from build123d import *

# Parameters (mm, degrees)
SKETCH1_R               = 21.25
SKETCH1_R_2             = 4.2
SKETCH1_R_3             = 2.9
BOSS_EXTRUDE1_DEPTH     = 2
CUT_EXTRUDE1_DEPTH      = 171.89177862
CUT_EXTRUDE1_DEPTH_BACK = 171.89177862
SKETCH2_W               = 15
SKETCH2_H               = 2


with BuildPart() as part:
    # Sketch1 → Boss-Extrude1 (new body)
    with BuildSketch(Plane.XY):
        Polygon((-158, -56), (-146.5, -56), (-146.5, -60), (-131.5, -60), (-131.5, -56), (-106.5, -56), (-106.5, -60), (-91.5, -60), (-91.5, -56), (-66.5, -56), (-66.5, -60), (-51.5, -60), (-51.5, -56), (-26.5, -56), (-26.5, -60), (-11.5, -60), (-11.5, -56), (11.5, -56), (11.5, -60), (26.5, -60), (26.5, -56), (51.5, -56), (51.5, -60), (66.5, -60), (66.5, -56), (91.5, -56), (91.5, -60), (106.5, -60), (106.5, -56), (131.5, -56), (131.5, -60), (146.5, -60), (146.5, -56), (158, -56), (158, -24), (160, -24), (160, -4), (158, -4), (158, 16), (160, 16), (160, 36), (158, 36), (158, 56), (146.5, 56), (146.5, 58), (131.5, 58), (131.5, 56), (106.5, 56), (106.5, 58), (91.5, 58), (91.5, 56), (66.5, 56), (66.5, 58), (51.5, 58), (51.5, 56), (26.5, 56), (26.5, 58), (11.5, 58), (11.5, 56), (-11.5, 56), (-11.5, 58), (-26.5, 58), (-26.5, 56), (-51.5, 56), (-51.5, 58), (-66.5, 58), (-66.5, 56), (-91.5, 56), (-91.5, 58), (-106.5, 58), (-106.5, 56), (-131.5, 56), (-131.5, 58), (-146.5, 58), (-146.5, 56), (-158, 56), (-158, 36), (-160, 36), (-160, 16), (-158, 16), (-158, -4), (-160, -4), (-160, -24), (-158, -24), align=None)
        with Locations((10.5, -18)):
            Circle(SKETCH1_R, mode=Mode.SUBTRACT)
        with Locations((-29, -18)):
            Circle(SKETCH1_R_2, mode=Mode.SUBTRACT)
        with Locations((50, -18)):
            Circle(SKETCH1_R_2, mode=Mode.SUBTRACT)
        with Locations((-125, -40)):
            Circle(SKETCH1_R_3, mode=Mode.SUBTRACT)
        with Locations((-71, -40)):
            Circle(SKETCH1_R_3, mode=Mode.SUBTRACT)
        with Locations((-125, 12)):
            Circle(SKETCH1_R_3, mode=Mode.SUBTRACT)
        with Locations((-71, 12)):
            Circle(SKETCH1_R_3, mode=Mode.SUBTRACT)
        with BuildLine():
            Line((-93.5, -14.916994756), (-93.5, -13.083005244))
            ThreePointArc((-93.5, -13.083005244), (-94.924535841, 8.581133525), (-107.310612225, -9.25))
            Line((-107.310612225, -9.25), (-112.7, -9.25))
            Line((-112.7, -9.25), (-112.7, -18.75))
            Line((-112.7, -18.75), (-107.310612225, -18.75))
            ThreePointArc((-107.310612225, -18.75), (-94.924535841, -36.581133525), (-93.5, -14.916994756))
        make_face(mode=Mode.SUBTRACT)
    extrude(amount=BOSS_EXTRUDE1_DEPTH)

    # Sketch2 → Cut-Extrude1 (cut, two sides: drawn at the far end of the back side and taken through both)
    with BuildSketch(Plane.XY.offset(2).offset(-CUT_EXTRUDE1_DEPTH_BACK)):
        with Locations((-139, 57)):
            Rectangle(SKETCH2_W, SKETCH2_H)
        with Locations((-99, 57)):
            Rectangle(SKETCH2_W, SKETCH2_H)
        with Locations((-59, 57)):
            Rectangle(SKETCH2_W, SKETCH2_H)
        with Locations((-19, 57)):
            Rectangle(SKETCH2_W, SKETCH2_H)
        with Locations((19, 57)):
            Rectangle(SKETCH2_W, SKETCH2_H)
        with Locations((59, 57)):
            Rectangle(SKETCH2_W, SKETCH2_H)
        with Locations((99, 57)):
            Rectangle(SKETCH2_W, SKETCH2_H)
        with Locations((139, 57)):
            Rectangle(SKETCH2_W, SKETCH2_H)
    extrude(amount=CUT_EXTRUDE1_DEPTH + CUT_EXTRUDE1_DEPTH_BACK, mode=Mode.SUBTRACT)


solid = part.part
Part model, mm, in its own coordinate system. Coordinates: 2 decimals unless noted, no trailing zeros. Loops run counter-clockwise (first coordinate to the right, second up) from the corner with the lowest first, then second, coordinate; pieces in that order, holes last. Notation, with made-up numbers: (72.5, -17) -> (91.5, -17) arc R11 ccw to (91.5, -10) -> close; hole circle Ø1 at (-15.75, -24). An arc over 180 degrees is marked (long way). Use a Markdown table: item, result. Add a question column.
Item 1: Band-saw the part on C-C on z = 1.3. Give the number of separate pieces and of enclosed holes in the cut face, plus the area to 3 significant figures.
Item 2: Probe probe 1 along Y at (x, z) = (-71, 0.9); probe 2 along X at (y, z) = (-34.5, 0.1); probe 3 along Y at (x, z) = (10.5, 1.45). List the from-to ranges inside material, lowest first.
Item 3: Band-saw the part on B-B on x = 75. Write the cut outline in (y, z).
Item 4: Flat gauge pins, fed straight in: P1, Ø1, axis at y = -57.5, z = 1, coming from the +X side; P2, Ø0.6, axis at y = -58, z = 1, coming from the -X side; P3, Ø0.6, axis at y = 10.5, z = 1, coming from the +X side. Where does each tip first touch, or does it go through?
Item 5: Pull direction Y, two halves, no side cores. Call faces 1 (the cylindrical face through (-73.1, 14, 1)), 2 (the flat face through (-2, 12, 2)): +Y half, -Y half, draft (parallel to the pull), parting line (faces both ways), or undercut.
Item 6: Band-saw the part on A-A on y = 12. Write the cut outline in (x, z).
Geometry says:
| question | item | result |
|---|---|---|
| 1 | separate pieces | 1 |
| 1 | enclosed holes | 8 |
| 1 | area | 33,500 mm² |
| 2 | probe 1 | -56 to -42.9, -37.1 to 9.1, 14.9 to 56 |
| 2 | probe 2 | -158 to -105.16, -90.84 to -2.89, 23.89 to 158 |
| 2 | probe 3 | -56 to -39.25, 3.25 to 56 |
| 3 | outline | (-56, 0) -> (56, 0) -> (56, 2) -> (-56, 2) -> close |
| 4 | P1 | x = 146.5 |
| 4 | P2 | x = -146.5 |
| 4 | P3 | x = 158 |
| 5 | face 1 | undercut |
| 5 | face 2 | draft |
| 6 | outline | (-158, 0) -> (-127.9, 0) -> (-127.9, 2) -> (-158, 2) -> close; (-122.1, 0) -> (-73.9, 0) -> (-73.9, 2) -> (-122.1, 2) -> close; (-68.1, 0) -> (158, 0) -> (158, 2) -> (-68.1, 2) -> close |
